Input: part model. Units: mm. Frame: model coordinates. Coordinates: 2 decimals unless noted, no trailing zeros. Order: outer loops, then holes, each group sorted by start corner. A loop starts at its lowest first (then second) coordinate and runs counter-clockwise, first axis right, second up. Notation, with made-up numbers: (-27, 10.5) -> (-5, 10.5) arc R28 cw to (-5, 35.5) -> close; hole circle Ø3 at (76, 49.25). An arc over 180 degrees is marked (long way). Write each question's results on one line, items separated by ' | '.
Autodesk Inventor part; units mm, degrees
ref_plane "YZ Plane" through (0, 0, 0) normal (1, 0, 0) x (0, 1, 0)
ref_plane "XZ Plane" through (0, 0, 0) normal (0, 1, 0) x (-1, 0, 0)
ref_plane "XY Plane" through (0, 0, 0) normal (0, 0, 1) x (1, 0, 0)
sketch "Sketch1" plane through (0, 0, 0) normal (1, 0, 0) x (0, 1, 0)
  line L0 (0, 0) -> (57.15, 0)
  line L1 (57.15, 0) -> (57.15, -254)
  line L2 (57.15, -254) -> (0, -254)
  line L3 (0, -254) -> (0, 0)
  dimension "d0" = 57.15
  dimension "d1" = 254
extrude "Extrusion1" add sketch "Sketch1" along normal blind 6.35
sketch "Sketch2" plane through (6.35, 0, 0) normal (1, 0, 0) x (0, 0, -1)
  line L0 (254, 57.15) -> (0, 57.15)
  circle A0 centre (209.55, 19.05) radius 5.9944
  line L1 (209.55, 19.05) -> (209.55, 26.0604)
  circle A1 centre (209.55, 26.0604) radius 15.494
  circle A2 centre (225.044, 26.0604) radius 1.4986
  circle A3 centre (217.297, 39.4786) radius 1.4986
  circle A4 centre (201.803, 39.4786) radius 1.4986
  circle A5 centre (194.056, 26.0604) radius 1.4986
  circle A6 centre (201.803, 12.6422) radius 1.4986
  circle A7 centre (217.297, 12.6422) radius 1.4986
  line L2 (209.55, 13.0556) -> (0, 13.0556)
  line L3 (0, 57.15) -> (0, 0)
  line L4 (0, 0) -> (254, 0)
  dimension "d7" = 11.9888
  dimension "d9" = 7.0104
  dimension "d10" = 30.988
  dimension "d11" = 2.9972
  dimension "d14" = 360
  dimension "d28" = 209.55
  dimension "d49" = 13.0556
extrude "Extrusion2" cut sketch "Sketch2" against normal through all contours A0 | A6 A1 L2 | L2 A1 A6 | A1 L2 A6 | A1 A6 L2 | A5 A1 | A1 A5 | A7 A1 | A1 A7 | A4 A1 | A1 A4 | A2 A1 | A1 A2 | A3 A1 | A1 A3
sketch "Sketch3" plane through (6.35, 0, 0) normal (1, 0, 0) x (0, 0, -1)
  circle A0 centre (209.55, 19.05) radius 5.9944
  circle A1 centre (201.803, 12.6422) radius 1.4986
  circle A2 centre (201.803, 39.4786) radius 1.4986
  circle A3 centre (225.044, 26.0604) radius 1.4986
  circle A4 centre (217.297, 39.4786) radius 1.4986
  circle A5 centre (194.056, 26.0604) radius 1.4986
  circle A6 centre (217.297, 12.6422) radius 1.4986
  line L0 (0, 57.15) -> (0, 0)
  line L1 (0, 0) -> (254, 0)
  line L2 (254, 0) -> (254, 57.15)
  line L3 (254, 57.15) -> (0, 57.15)
  line L4 (209.55, 19.05) -> (127, 19.05)
  circle A7 centre (127, 19.05) radius 14.9225
  circle A8 centre (127, 19.05) radius 36.5125
  line L5 (127, 19.05) -> (44.45, 19.05)
  circle A9 centre (44.45, 19.05) radius 14.9225
  dimension "d18" = 82.55
  dimension "d19" = 29.845
  dimension "d27" = 73.025
  dimension "d29" = 82.55
  dimension "d30" = 29.845
extrude "Extrusion3" cut sketch "Sketch3" against normal through all contours A9 | A7 L5 L4 | L4 L5 A7
sketch "Sketch4" plane through (6.35, 0, 0) normal (1, 0, 0) x (0, 0, -1)
  line L0 (0, 57.15) -> (0, 0)
  line L1 (254, 0) -> (254, 57.15)
  line L2 (0, 57.15) -> (6.35, 57.15)
  line L3 (6.35, 57.15) -> (18.35, 57.15)
  line L4 (18.35, 57.15) -> (18.35, 49.15)
  circle A0 centre (18.35, 49.15) radius 2.1
  line L5 (6.35, 0) -> (18.35, 0)
  line L6 (18.35, 0) -> (18.35, 8)
  circle A1 centre (18.35, 8) radius 2.1
  line L7 (254, 57.15) -> (247.65, 57.15)
  line L8 (247.65, 57.15) -> (235.65, 57.15)
  line L9 (247.65, 0) -> (235.65, 0)
  circle A2 centre (235.65, 49.15) radius 2.1
  circle A3 centre (235.65, 8) radius 2.1
  line L10 (254, 57.15) -> (0, 57.15)
  dimension "d31" = 6.35
  dimension "d32" = 12
  dimension "d33" = 8
  dimension "d34" = 4.2
  dimension "d35" = 12
  dimension "d36" = 8
  dimension "d37" = 4.2
  dimension "d38" = 6.35
  dimension "d39" = 12
  dimension "d41" = 12
  dimension "d43" = 4.2
  dimension "d44" = 4.2
  dimension "d45" = 6.35
  dimension "d46" = 6.35
extrude "Extrusion4" cut sketch "Sketch4" against normal through all
properties part number "DriveRail"
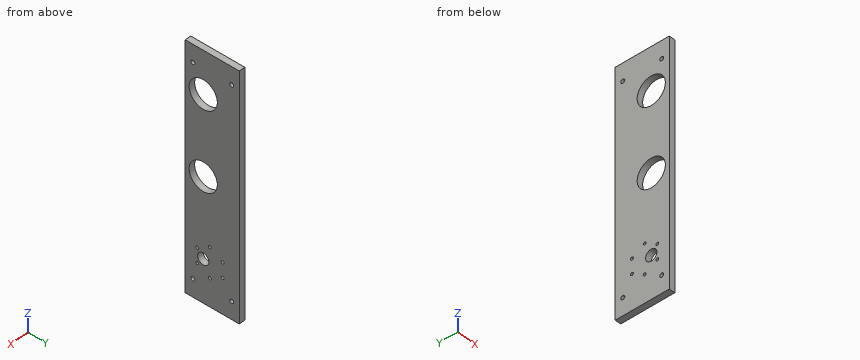
(1) Cut plane C-C, the plane z = -235.65. Return loops of the section in (x, y).
Return value:
outline: (0, 0) -> (6.35, 0) -> (6.35, 5.9) -> (0, 5.9) -> close; (0, 10.1) -> (6.35, 10.1) -> (6.35, 47.05) -> (0, 47.05) -> close; (0, 51.25) -> (6.35, 51.25) -> (6.35, 57.15) -> (0, 57.15) -> close
(2) Pin query (flat end, axial travel): P1, Ø5, axis at y = 39.48, z = -217.3, coming from the +X side. Return the tip coordinate at first contact, or that it passes through.
Return value:
P1: x = 6.35
(3) Cut plane D-D, the plane x = 3. Count the separate pieces of the cut face and the enclosed holes in it, plus the area to 3 significant figures.
Return value:
separate pieces: 1 | enclosed holes: 13 | area: 12,900 mm2
(4) Cut plane B-B, the plane z = -44.45. Return loops of the section in (x, y).
Return value:
outline: (0, 0) -> (6.35, 0) -> (6.35, 4.13) -> (0, 4.13) -> close; (0, 33.97) -> (6.35, 33.97) -> (6.35, 57.15) -> (0, 57.15) -> close
(5) Line query: line 1 along Y through (x, z) = (3, -235.65); line 2 along Z through (x, y) = (2, 18.5); line 3 along Y through (x, z) = (2, -44.45). Output: solid intervals per line, ascending. Write a range as from..to.
Return value:
line 1: 0..5.9, 10.1..47.05, 51.25..57.15 | line 2: -254..-215.52, -203.58..-141.91, -112.09..-59.36, -29.54..0 | line 3: 0..4.13, 33.97..57.15
(6) Cut plane A-A, the plane y = 19.05. Return loops of the section in (x, z), plus the area to 3 significant figures.
Return value:
outline: (0, -254) -> (6.35, -254) -> (6.35, -215.54) -> (0, -215.54) -> close; (0, -203.56) -> (6.35, -203.56) -> (6.35, -141.92) -> (0, -141.92) -> close; (0, -112.08) -> (6.35, -112.08) -> (6.35, -59.37) -> (0, -59.37) -> close; (0, -29.53) -> (6.35, -29.53) -> (6.35, 0) -> (0, 0) -> close | area: 1,160 mm2
